```python
from build123d import *

# Parameters (mm, degrees)
EXTRUDE_1_DEPTH                  = 35
CUT_EXTRUDE_1_DEPTH              = 30
SKETCH_4_R                       = 15
CUT_EXTRUDE_3_DEPTH              = 10
SKETCH_9_R                       = 6.5
CUT_EXTRUDE_6_DEPTH              = 5
CUT_EXTRUDE_8_REACH              = 183.675
SKETCH_12_R                      = 1.2
CUT_EXTRUDE_9_DEPTH              = 5
CUT_EXTRUDE_10_REACH             = 7
SKETCH_14_R                      = 1.7
SKETCH_15_R                      = 1.7
CUT_EXTRUDE_11_DEPTH             = 5
SKETCH_21_R                      = 6
EXTRUDE_7_DEPTH                  = 25
FILLET_1_R                       = 10
FILLET_2_R                       = 10
FILLET_3_R                       = 10
CUT_EXTRUDE_17_REACH             = 7
SKETCH_23_R                      = 2.25
SKETCH_24_R                      = 2.25
CUT_EXTRUDE_18_DEPTH             = 36
HOLE_WIZARD_M4_1_D               = 3.3
HOLE_WIZARD_M4_1_DEPTH           = 11.5
HOLE_WIZARD_M4_1_TIP             = 0.991420021
CUT_EXTRUDE_19_REACH             = 37
SKETCH_3_R                       = 15
CUT_EXTRUDE_19_DIRECTION_2_DEPTH = 1
HOLE_WIZARD_M4_2_D               = 3.3
HOLE_WIZARD_M4_2_DEPTH           = 11.5
HOLE_WIZARD_M4_2_TIP             = 0.991420021


with BuildPart() as part:
    # 스케치1 → 보스-돌출1 (new body)
    with BuildSketch(Plane(origin=(0, 0, 0), x_dir=(1, 0, 0), z_dir=(0, 1, 0))):
        with BuildLine():
            Line((-35.5, 121.9), (10, 121.9))
            Line((10, 121.9), (58.5, 121.9))
            ThreePointArc((58.5, 121.9), (65.217514421, 119.117514421), (68, 112.4))
            Line((68, 112.4), (68, 51.135104302))
            ThreePointArc((68, 51.135104302), (71.192111556, 41.884495106), (79.409836066, 36.571082779))
            ThreePointArc((79.409836066, 36.571082779), (94.419473689, 32.440718825), (109.185841564, 27.510860028))
            ThreePointArc((109.185841564, 27.510860028), (136.08110305, -30.166214357), (78.404028665, -57.061475843))
            ThreePointArc((78.404028665, -57.061475843), (44.729635533, -48.038449398), (10, -45))
            Line((10, -45), (-35, -45))
            ThreePointArc((-35, -45), (-42.071067812, -42.071067812), (-45, -35))
            Line((-45, -35), (-45, 112.4))
            ThreePointArc((-45, 112.4), (-42.217514421, 119.117514421), (-35.5, 121.9))
        make_face()
    extrude(amount=EXTRUDE_1_DEPTH)

    # 스케치2 → 컷-돌출1 (cut)
    with BuildSketch(Plane(origin=(0, 35, 0), x_dir=(1, 0, 0), z_dir=(0, 1, 0))):
        with BuildLine():
            Line((-40, 112.4), (-40, -35))
            ThreePointArc((-40, -35), (-38.535533906, -38.535533906), (-35, -40))
            Line((-35, -40), (10, -40))
            ThreePointArc((10, -40), (45.597876422, -43.114410632), (80.114129382, -52.363012739))
            ThreePointArc((80.114129382, -52.363012739), (131.382639946, -28.45611364), (107.475740848, 22.812396924))
            ThreePointArc((107.475740848, 22.812396924), (92.963965522, 27.657258155), (78.213114754, 31.716408938))
            ThreePointArc((78.213114754, 31.716408938), (67.256148741, 38.800958708), (63, 51.135104302))
            Line((63, 51.135104302), (63, 112.4))
            ThreePointArc((63, 112.4), (61.681980515, 115.581980515), (58.5, 116.9))
            Line((58.5, 116.9), (-35.5, 116.9))
            ThreePointArc((-35.5, 116.9), (-38.681980515, 115.581980515), (-40, 112.4))
        make_face()
    extrude(amount=-CUT_EXTRUDE_1_DEPTH, mode=Mode.SUBTRACT)

    # 스케치4 → 컷-돌출3 (cut)
    with BuildSketch(Plane.ZY.offset(45)):
        with Locations((0, 35)):
            Circle(SKETCH_4_R)
    extrude(amount=-CUT_EXTRUDE_3_DEPTH, mode=Mode.SUBTRACT)

    # 스케치9 → 컷-돌출6 (cut)
    with BuildSketch(Plane.ZY.offset(45)):
        with Locations((-71.4, 35)):
            Circle(SKETCH_9_R)
    extrude(amount=-CUT_EXTRUDE_6_DEPTH, mode=Mode.SUBTRACT)

    # 스케치12 → 컷-돌출8 (cut, up to next)
    with BuildSketch(Plane(origin=(0, 0, -121.9), x_dir=(-1, 0, 0), z_dir=(0, 0, -1)), mode=Mode.PRIVATE) as cut_extrude_8_sk1:
        with Locations((-44, 25)):
            Circle(SKETCH_12_R)
    cut_extrude_8_tool1 = extrude(cut_extrude_8_sk1.sketch, amount=-CUT_EXTRUDE_8_REACH, mode=Mode.PRIVATE) & part.part
    add(cut_extrude_8_tool1.solids().sort_by_distance((44, 25, -121.9))[0], mode=Mode.SUBTRACT)
    # 스케치12 → 컷-돌출8 (cut, up to next)
    with BuildSketch(Plane(origin=(0, 0, -121.9), x_dir=(-1, 0, 0), z_dir=(0, 0, -1)), mode=Mode.PRIVATE) as cut_extrude_8_sk2:
        with Locations((-28, 25)):
            Circle(SKETCH_12_R)
    cut_extrude_8_tool2 = extrude(cut_extrude_8_sk2.sketch, amount=-CUT_EXTRUDE_8_REACH, mode=Mode.PRIVATE) & part.part
    add(cut_extrude_8_tool2.solids().sort_by_distance((28, 25, -121.9))[0], mode=Mode.SUBTRACT)

    # 스케치13 → 컷-돌출9 (cut)
    with BuildSketch(Plane(origin=(0, 35, 0), x_dir=(1, 0, 0), z_dir=(0, 1, 0))):
        with BuildLine():
            Line((-42, -35), (-42, -28.086909805))
            Line((-42, -28.086909805), (-42, 64.9))
            Line((-42, 64.9), (-42, 77.9))
            Line((-42, 77.9), (-42, 112.4))
            ThreePointArc((-42, 112.4), (-40.096194078, 116.996194078), (-35.5, 118.9))
            Line((-35.5, 118.9), (58.5, 118.9))
            ThreePointArc((58.5, 118.9), (63.096194078, 116.996194078), (65, 112.4))
            Line((65, 112.4), (65, 51.135104302))
            ThreePointArc((65, 51.135104302), (68.830533867, 40.034373267), (78.691803279, 33.658278474))
            ThreePointArc((78.691803279, 33.658278474), (93.546168789, 29.570642423), (108.159781134, 24.691782166))
            ThreePointArc((108.159781134, 24.691782166), (133.262025188, -29.140153927), (79.430089095, -54.24239798))
            ThreePointArc((79.430089095, -54.24239798), (45.250580066, -45.084026139), (10, -42))
            Line((10, -42), (-35, -42))
            ThreePointArc((-35, -42), (-39.949747468, -39.949747468), (-42, -35))
        make_face()
        with BuildLine():
            Line((-40, -28.086909805), (-40, -35))
            ThreePointArc((-40, -35), (-38.535533906, -38.535533906), (-35, -40))
            Line((-35, -40), (10, -40))
            ThreePointArc((10, -40), (45.597876422, -43.114410632), (80.114129382, -52.363012739))
            ThreePointArc((80.114129382, -52.363012739), (131.382639946, -28.45611364), (107.475740848, 22.812396924))
            ThreePointArc((107.475740848, 22.812396924), (92.963965522, 27.657258155), (78.213114754, 31.716408938))
            ThreePointArc((78.213114754, 31.716408938), (67.256148741, 38.800958708), (63, 51.135104302))
            Line((63, 51.135104302), (63, 112.4))
            ThreePointArc((63, 112.4), (61.681980515, 115.581980515), (58.5, 116.9))
            Line((58.5, 116.9), (-35.5, 116.9))
            ThreePointArc((-35.5, 116.9), (-38.681980515, 115.581980515), (-40, 112.4))
            Line((-40, 112.4), (-40, 77.9))
            Line((-40, 77.9), (-40, 64.9))
            Line((-40, 64.9), (-40, -28.086909805))
        make_face(mode=Mode.SUBTRACT)
    extrude(amount=-CUT_EXTRUDE_9_DEPTH, mode=Mode.SUBTRACT)

    # 스케치14 → 컷-돌출10 (cut, up to next)
    with BuildSketch(Plane(origin=(0, 5, 0), x_dir=(1, 0, 0), z_dir=(0, 1, 0)), mode=Mode.PRIVATE) as cut_extrude_10_sk1:
        with Locations((36, 53.65)):
            Circle(SKETCH_14_R)
    cut_extrude_10_tool1 = extrude(cut_extrude_10_sk1.sketch, amount=-CUT_EXTRUDE_10_REACH, mode=Mode.PRIVATE) & part.part
    add(cut_extrude_10_tool1.solids().sort_by_distance((36, 5, -53.65))[0], mode=Mode.SUBTRACT)
    # 스케치14 → 컷-돌출10 (cut, up to next)
    with BuildSketch(Plane(origin=(0, 5, 0), x_dir=(1, 0, 0), z_dir=(0, 1, 0)), mode=Mode.PRIVATE) as cut_extrude_10_sk2:
        with Locations((28, 53.65)):
            Circle(SKETCH_14_R)
    cut_extrude_10_tool2 = extrude(cut_extrude_10_sk2.sketch, amount=-CUT_EXTRUDE_10_REACH, mode=Mode.PRIVATE) & part.part
    add(cut_extrude_10_tool2.solids().sort_by_distance((28, 5, -53.65))[0], mode=Mode.SUBTRACT)
    # 스케치14 → 컷-돌출10 (cut, up to next)
    with BuildSketch(Plane(origin=(0, 5, 0), x_dir=(1, 0, 0), z_dir=(0, 1, 0)), mode=Mode.PRIVATE) as cut_extrude_10_sk3:
        with Locations((44, 53.65)):
            Circle(SKETCH_14_R)
    cut_extrude_10_tool3 = extrude(cut_extrude_10_sk3.sketch, amount=-CUT_EXTRUDE_10_REACH, mode=Mode.PRIVATE) & part.part
    add(cut_extrude_10_tool3.solids().sort_by_distance((44, 5, -53.65))[0], mode=Mode.SUBTRACT)

    # 스케치15 → 컷-돌출11 (cut)
    with BuildSketch(Plane.XZ):
        with Locations((-34, -65.4)):
            Circle(SKETCH_15_R)
        with Locations((-34, -71.4)):
            Circle(SKETCH_15_R)
        with Locations((-34, -77.4)):
            Circle(SKETCH_15_R)
    extrude(amount=-CUT_EXTRUDE_11_DEPTH, mode=Mode.SUBTRACT)

    # 스케치21 → 보스-돌출7 (add)
    with BuildSketch(Plane(origin=(0, 5, 0), x_dir=(1, 0, 0), z_dir=(0, 1, 0))):
        with Locations((-35, 111.9)):
            Circle(SKETCH_21_R)
        with Locations((-15, -35)):
            Circle(SKETCH_21_R)
        with Locations((-35, 45)):
            Circle(SKETCH_21_R)
        with Locations((63.320185927, 35.717422309)):
            Circle(SKETCH_21_R)
        with Locations((46.46611731, -38.190371867)):
            Circle(SKETCH_21_R)
    extrude(amount=EXTRUDE_7_DEPTH)

    # 필렛1
    fillet_1_edges = [part.edges().sort_by_distance(p)[0] for p in [
        (-40, 17.5, -108.58337521),
        (-31.68337521, 17.5, -116.9),
        (69.25374262, 17.5, -36.60787442),
        (65.60491959, 17.5, -41.265394199),
        (42.366311792, 17.5, 42.571193105),
        (48.820345194, 17.5, 43.709213328),
    ]]
    fillet(fillet_1_edges, radius=FILLET_1_R)

    # 필렛2
    fillet_2_edges = [part.edges().sort_by_distance(p)[0] for p in [
        (-40, 17.5, -48.31662479),
        (-40, 17.5, -41.68337521),
    ]]
    fillet(fillet_2_edges, radius=FILLET_2_R)

    # 필렛3
    fillet_3_edges = [part.edges().sort_by_distance(p)[0] for p in [
        (-18.31662479, 17.5, 40),
        (-11.68337521, 17.5, 40),
    ]]
    fillet(fillet_3_edges, radius=FILLET_3_R)

    # 스케치23 → 컷-돌출17 (cut, up to next)
    with BuildSketch(Plane(origin=(0, 5, 0), x_dir=(1, 0, 0), z_dir=(0, 1, 0)), mode=Mode.PRIVATE) as cut_extrude_17_sk1:
        with Locations((12, 0)):
            Circle(SKETCH_23_R)
    cut_extrude_17_tool1 = extrude(cut_extrude_17_sk1.sketch, amount=-CUT_EXTRUDE_17_REACH, mode=Mode.PRIVATE) & part.part
    add(cut_extrude_17_tool1.solids().sort_by_distance((12, 5, 0))[0], mode=Mode.SUBTRACT)
    # 스케치23 → 컷-돌출17 (cut, up to next)
    with BuildSketch(Plane(origin=(0, 5, 0), x_dir=(1, 0, 0), z_dir=(0, 1, 0)), mode=Mode.PRIVATE) as cut_extrude_17_sk2:
        with Locations((12, -8)):
            Circle(SKETCH_23_R)
    cut_extrude_17_tool2 = extrude(cut_extrude_17_sk2.sketch, amount=-CUT_EXTRUDE_17_REACH, mode=Mode.PRIVATE) & part.part
    add(cut_extrude_17_tool2.solids().sort_by_distance((12, 5, 8))[0], mode=Mode.SUBTRACT)
    # 스케치23 → 컷-돌출17 (cut, up to next)
    with BuildSketch(Plane(origin=(0, 5, 0), x_dir=(1, 0, 0), z_dir=(0, 1, 0)), mode=Mode.PRIVATE) as cut_extrude_17_sk3:
        with Locations((12, 8)):
            Circle(SKETCH_23_R)
    cut_extrude_17_tool3 = extrude(cut_extrude_17_sk3.sketch, amount=-CUT_EXTRUDE_17_REACH, mode=Mode.PRIVATE) & part.part
    add(cut_extrude_17_tool3.solids().sort_by_distance((12, 5, -8))[0], mode=Mode.SUBTRACT)

    # 스케치24 → 컷-돌출18 (cut, through all)
    with BuildSketch(Plane.XZ):
        with Locations((-34, -8)):
            Circle(SKETCH_24_R)
        with Locations((-34, 0)):
            Circle(SKETCH_24_R)
        with Locations((-34, 8)):
            Circle(SKETCH_24_R)
    extrude(amount=-CUT_EXTRUDE_18_DEPTH, mode=Mode.SUBTRACT)

    # M4 나사 구멍1
    with Locations(Plane(origin=(0, 30, 0), x_dir=(1, 0, 0), z_dir=(0, 1, 0))):
        with Locations((-35, 111.9), (-35, 45), (-15, -35), (46.46611731, -38.190371867), (63.320185927, 35.717422309)):
            Hole(HOLE_WIZARD_M4_1_D / 2, depth=HOLE_WIZARD_M4_1_DEPTH)
            with Locations((0, 0, -(HOLE_WIZARD_M4_1_DEPTH + HOLE_WIZARD_M4_1_TIP / 2))):  # 118° drill point
                Cone(0, HOLE_WIZARD_M4_1_D / 2, HOLE_WIZARD_M4_1_TIP, mode=Mode.SUBTRACT)

    # 스케치3 → 컷-돌출19 (cut, up to next)
    with BuildSketch(Plane.XZ, mode=Mode.PRIVATE) as cut_extrude_19_sk1:
        with Locations((93.794935115, 14.775307907)):
            Circle(SKETCH_3_R)
    cut_extrude_19_tool1 = extrude(cut_extrude_19_sk1.sketch, amount=-CUT_EXTRUDE_19_REACH, mode=Mode.PRIVATE) & part.part
    add(cut_extrude_19_tool1.solids().sort_by_distance((93.794935, 0, 14.775308))[0], mode=Mode.SUBTRACT)

    # 스케치3 → 컷-돌출19 direction 2 (cut)
    with BuildSketch(Plane.XZ):
        with Locations((93.794935115, 14.775307907)):
            Circle(SKETCH_3_R)
    extrude(amount=CUT_EXTRUDE_19_DIRECTION_2_DEPTH, mode=Mode.SUBTRACT)

    # M4 나사 구멍2
    with Locations(Plane(origin=(0, 5, 0), x_dir=(1, 0, 0), z_dir=(0, 1, 0))):
        with Locations((46.810304075, 2.325699259), (101.319378268, 5.89792975), (112.588787531, -21.615710774), (86.270491962, -35.448545565)):
            Hole(HOLE_WIZARD_M4_2_D / 2, depth=HOLE_WIZARD_M4_2_DEPTH)
            with Locations((0, 0, -(HOLE_WIZARD_M4_2_DEPTH + HOLE_WIZARD_M4_2_TIP / 2))):  # 118° drill point
                Cone(0, HOLE_WIZARD_M4_2_D / 2, HOLE_WIZARD_M4_2_TIP, mode=Mode.SUBTRACT)


solid = part.part
```
Work out the finished part from the listing and answer in its coordinate system (mm). A direction names the side the tool comes from. Coordinates: 2 decimals unless noted, no trailing zeros. Loops run counter-clockwise (first coordinate to the right, second up) from the corner with the lowest first, then second, coordinate; pieces in that order, holes last. Notation, with made-up numbers: (53, -19.5) - (80, -19.5) arc R29 ccw to (80, 11.5) - close; hole circle Ø6 at (10, 57.25). An arc over 180 degrees is marked (long way). Use a Markdown table: item, result.
Item 1: Given pin 1 Ø2.5 at (x, z) = (12, -8) entering from +Y; pin 2 Ø4 at (x, z) = (44, -53.65) entering from +Y; pin 3 Ø1.4 at (x, y) = (28, 25) entering from +Z; pin 4 Ø6 at (x, y) = (1.5, 9.5) entering from +Z, each flat-ended and moving along its own axis, determine where each tip first touches the part or whether it passes through.
Evaluation:
| item | result |
|---|---|
| pin 1 | passes through |
| pin 2 | stops at y = 5 |
| pin 3 | stops at z = 45.88 |
| pin 4 | stops at z = 45 |
Item 2: Consider probe 1 along X at (y, z) = (28, -86); probe 2 along X at (y, z) = (21.5, -111.9); probe 3 along Z at (x, y) = (-35, 27.5). Determine where each line is inside the solid, lowest interval first. Write a range as from..to.
Evaluation:
| item | result |
|---|---|
| probe 1 | x = -45..-40, 63..68 |
| probe 2 | x = -45..-36.65, -33.35..-28.46, 63..68 |
| probe 3 | z = -121.9..-113.55, -110.25..-105.36, -51.54..-46.65, -43.35..-38.46, 40..45 |
Item 3: Find section A-A, the plane x = 20. Determine the outline of the cut face in (y, z).
Evaluation:
| item | result |
|---|---|
| outline | (0, -121.9) - (35, -121.9) - (35, -118.9) - (30, -118.9) - (30, -116.9) - (5, -116.9) - (5, 40.24) - (30, 40.24) - (30, 42.25) - (35, 42.25) - (35, 45.25) - (0, 45.25) - close |
Item 4: For faces 5 (the cylindrical face through (-31.854, 2.465, 8.676)), 6 (the cylindrical face through (-43, 20, 0)), 7 (the flat face through (68, 17, -82)), 8 (the flat face through (-42, 33, -40)), determine the directions among +Z, -Z, +X, -X, +Y, -Y from which every point of the face is accessible in a straight line to the end or side of a thin tool.
Evaluation:
| item | result |
|---|---|
| face 5 | +Y, -Y |
| face 6 | -X, +Y |
| face 7 | -Z, +X, +Y, -Y |
| face 8 | +Y |
Item 5: The mould has two halves that part along X. Classify faces 1 (the cylindrical face through (71.11, 17.26, -41.99)), 2 (the cylindrical face through (-39.9, 32.5, 40)), 3 (the cylindrical face through (78.81, 2.46, 15.43)), 4 (the flat face through (11, 17, -121.9)): +X half, -X half, draft (parallel to the pull), parting line (faces both ways), or undercut.
Evaluation:
| item | result |
|---|---|
| face 1 | +X half |
| face 2 | undercut |
| face 3 | undercut |
| face 4 | draft |
